Study the drawing (mm; zero at the part's minimum x, y, z) and answer. A direction names the side the tool comes from. Round coordinates to 2 decimals unless told otherwise and drop trailing zeros. Write each loop counter-clockwise with the first axis right and the second up, starting at its lowest first coordinate (ties: lowest second). Pieces come first, ordered by that corner, then holes.
(1) A cutting plane is placed at A-A, the plane x = 19.05. Give the vertices of the cut face in (y, z), and give its area (3 significant figures).
(2) The mould has two halves that part along X. Classify the marked faces 4, 5 and 6: +X half, -X half, draft (parallel to the pull), parting line (faces both ways), or undercut.
(3) Each of these flat-tipped pins is pushed along its axis until it touches: pin 1 Ø9.5 at (x, y) = (32, 22) entering from +Z; pin 2 Ø1.5 at (x, y) = (57.5, 9) entering from -Z; pin 3 Ø10 at (y, z) = (14, 28.5) entering from +X; pin 4 Ø7 at (y, z) = (25, 3.5) entering from -X. Where does it stop, or does it pass through?
(4) For the marked faces 1, 2 and 3, determine the directions among +Z, -Z, +X, -X, +Y, -Y from which every point of the face is accessible in a straight line to the end or side of a thin tool.
(5) A cutting plane is placed at D-D, the plane x = 36. Give the vertices of the cut face in (y, z), and give its area (3 significant figures).
(6) A cutting plane is placed at B-B, the plane z = 50.8. Give the vertices of the cut face in (x, y), and give its area (3 significant figures).
(7) Find the intervals of material crossed by probe 1 along Z at (x, y) = (19.05, 41); probe 2 along Y at (x, z) = (48, 40); probe 3 along X at (y, z) = (50, 50), in increasing order.
(8) A cutting plane is placed at C-C, the plane y = 18. Give the vertices of the cut face in (x, z), and give its area (3 significant figures).
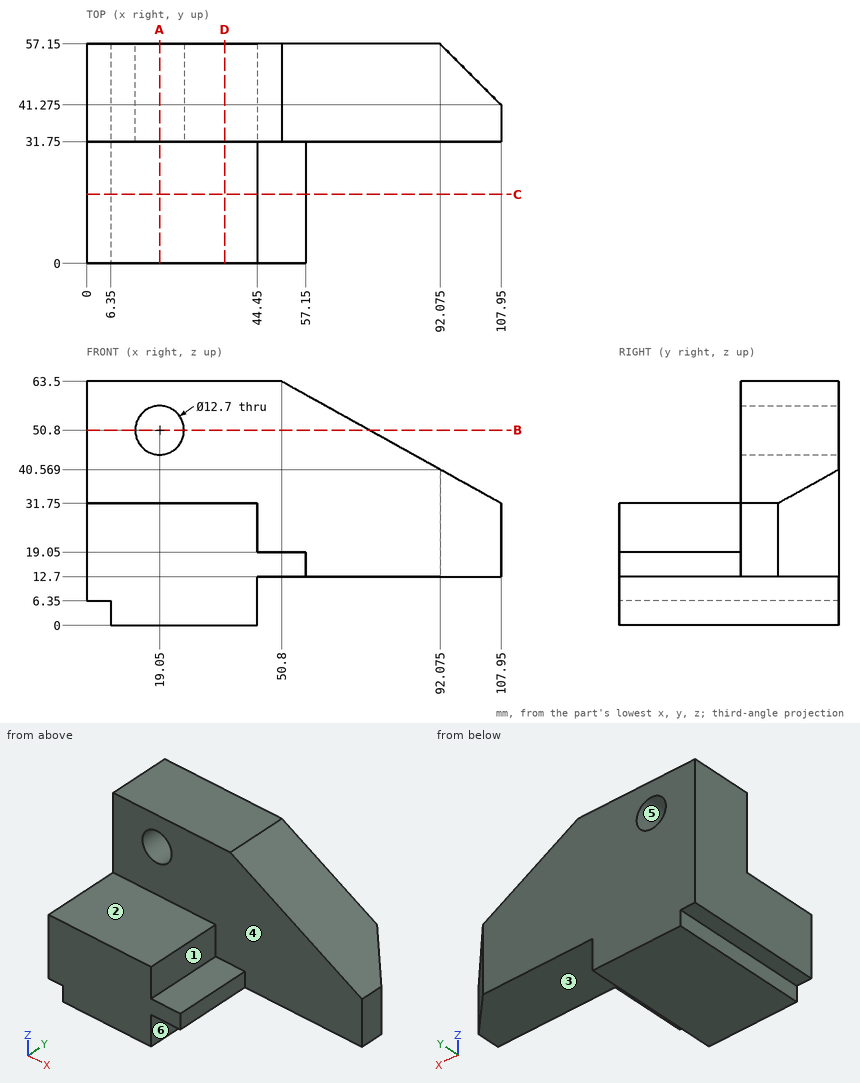
Solutions:
1. outline: (0, 0) - (57.15, 0) - (57.15, 44.45) - (31.75, 44.45) - (31.75, 31.75) - (0, 31.75) - close; (31.75, 57.15) - (57.15, 57.15) - (57.15, 63.5) - (31.75, 63.5) - close
1. area: 2,300 mm2
2. face 4: draft
2. face 5: undercut
2. face 6: +X half
3. pin 1: stops at z = 31.75
3. pin 2: stops at z = 12.7
3. pin 3: stops at x = 44.45
3. pin 4: stops at x = 0
4. face 1: +Z, +X, -Y
4. face 2: +Z, +X, -X, -Y
4. face 3: -Z, +X, +Y, -Y
5. outline: (0, 0) - (57.15, 0) - (57.15, 63.5) - (31.75, 63.5) - (31.75, 31.75) - (0, 31.75) - close
5. area: 2,620 mm2
6. outline: (0, 31.75) - (12.7, 31.75) - (12.7, 57.15) - (0, 57.15) - close; (25.4, 31.75) - (73.66, 31.75) - (73.66, 57.15) - (25.4, 57.15) - close
6. area: 1,550 mm2
7. probe 1: z = 0 to 44.45, 57.15 to 63.5
7. probe 2: y = 31.75 to 57.15
7. probe 3: x = 0 to 12.75, 25.35 to 75.1
8. outline: (0, 6.35) - (6.35, 6.35) - (6.35, 0) - (44.45, 0) - (44.45, 12.7) - (57.15, 12.7) - (57.15, 19.05) - (44.45, 19.05) - (44.45, 31.75) - (0, 31.75) - close
8. area: 1,450 mm2
